Could you check a few things on this model? Use its own coordinates, in mm. Face numbers are marked on the shaded views. Give positions to 0.01 mm unless a question says otherwise; leave off trailing zeros. Order: outer loops, then holes, each group sorted by start corner. A loop starts at its lowest first (then second) coordinate and runs counter-clockwise, first axis right, second up. Notation, with made-up numbers: M 20,69.25 L 27,69.25 A25 ccw 27,88.25 Z; hole C -33,81.25 d11. An arc over 180 degrees is marked long. Answer in a Markdown table with one row per item. Add a question column.
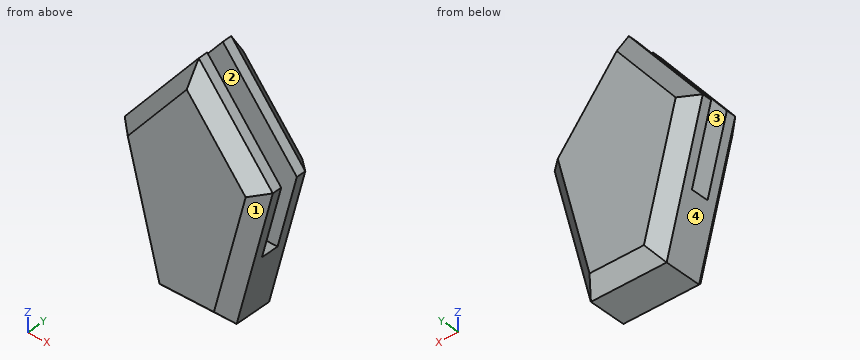
```python
from build123d import *

# Parameters (mm, degrees)
F1_DEPTH = 4.7
F2_W     = 1.3
F2_H     = 12
F3_DEPTH = 10
F4_SIZE  = 1


with BuildPart() as f1:
    # F0 (on Front) → F1 (new body)
    with BuildSketch(Plane.XZ):
        Polygon((-5.37627, 10.166253), (-2.75, 0), (2.75, 0), (5.37627, 10.166253), (0, 16.75), align=None)
    extrude(amount=F1_DEPTH)

    # F2 (on Right) → F3 (cut, symmetric)
    with BuildSketch(Plane.YZ):
        with Locations((-2.35, 10.75)):
            Rectangle(F2_W, F2_H)
    extrude(amount=F3_DEPTH, both=True, mode=Mode.SUBTRACT)

    # F4
    f4_edges = [f1.edges().sort_by_distance(p)[0] for p in [
        (-4.063135, -4.7, 5.083127),
        (0, -4.7, 0),
        (4.063135, -4.7, 5.083127),
        (2.688135, -4.7, 13.458127),
        (-2.688135, -4.7, 13.458127),
        (-4.063135, 0, 5.083127),
        (0, 0, 0),
        (4.063135, 0, 5.083127),
        (2.688135, 0, 13.458127),
        (-2.688135, 0, 13.458127),
    ]]
    chamfer(f4_edges, length=F4_SIZE)


solid = f1.part
```
1. Will these pins go through, and if not, where does the flat tip stop? P1, Ø0.6, axis at x = 2, y = -2.5, coming from the +Z side; P2, Ø2, axis at y = -1, z = 14.5, coming from the -X side.
2. If I drill on line 1 along Y through (x, z) = (3, 10.5); line 2 along Z through (x, y) = (-2, -2.2); line 3 along Y through (x, z) = (-4, 6.75), over which ranges is the centre line in solid material (lowest first)? Write a range as [from, to].
3. Suppose I cut it at A-A on z = 5.5. List the corners of the cut face in (x, y) for me.
4. Suppose I cut it at D-D on z = 15.5. List the corners of the cut face in (x, y) for me.
5. Suppose I cut it at C-C on y = -0.35. List the corners of the cut face in (x, z) for me.
6. Suppose I cut it at B-B on x = 1.75. List the corners of the cut face in (y, z) for me, plus the area to 3 significant figures.
7. Thinking about a two-plate mould opening in Y: for the marked faces 1, 2, 3 and 4, which applies, pulls with the +Y half, pulls with the -Y half, needs draft (parallel to the pull), parting line crosses it, or undercut?
Findings below:
| question | item | result |
|---|---|---|
| 1 | P1 | z = 4.75 |
| 1 | P2 | x = -2.65 |
| 2 | line 1 | [-4.7, -3], [-1.7, 0] |
| 2 | line 2 | [0, 4.75] |
| 2 | line 3 | [-4.18, -3], [-1.7, -0.52] |
| 3 | outline | M -4.17,-3.7 L -3.14,-4.7 L 3.14,-4.7 L 4.17,-3.7 L 4.17,-3 L -4.17,-3 Z; M -4.17,-1.7 L 4.17,-1.7 L 4.17,-1 L 3.14,0 L -3.14,0 L -4.17,-1 Z |
| 4 | outline | M -1.02,-3.7 L 0,-4.49 L 1.02,-3.7 L 1.02,-3 L -1.02,-3 Z; M -1.02,-1.7 L 1.02,-1.7 L 1.02,-1 L 0,-0.21 L -1.02,-1 Z |
| 5 | outline | M -4.66,10.01 L -2.25,0.65 L 2.25,0.65 L 4.66,10.01 L 0,15.72 Z |
| 6 | outline | M -4.7,1 L -3.7,0 L -1,0 L 0,1 L 0,13.03 L -1,14.61 L -1.7,14.61 L -1.7,4.75 L -3,4.75 L -3,14.61 L -3.7,14.61 L -4.7,13.03 Z |
| 6 | area | 53.3 mm2 |
| 7 | face 1 | pulls with the -Y half |
| 7 | face 2 | undercut |
| 7 | face 3 | undercut |
| 7 | face 4 | needs draft |
